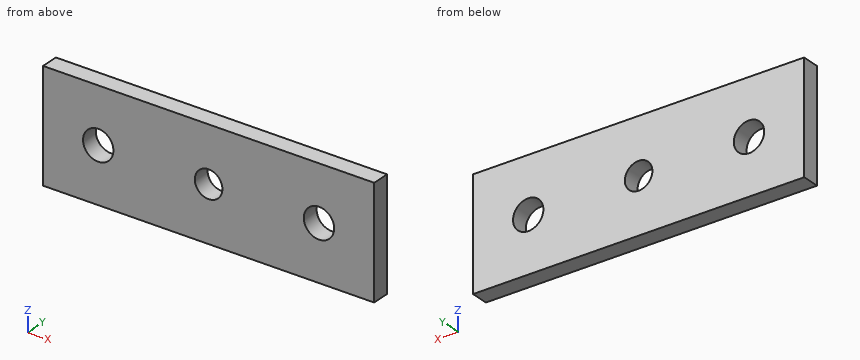
```python
from build123d import *

# Parameters (mm, degrees)
SKETCH1_W             = 60
SKETCH1_H             = 20
BOSS_EXTRUDE1_DEPTH   = 3.175
SKETCH4_R             = 2.75
CUT_EXTRUDE1_DEPTH    = 3.175
M6X1_0_TAPPED_HOLE1_D = 5


with BuildPart() as part:
    # Sketch1 → Boss-Extrude1 (new body)
    with BuildSketch(Plane(origin=(0, 0, 0), x_dir=(1, 0, 0), z_dir=(0, 1, 0))):
        with Locations((30, 10)):
            Rectangle(SKETCH1_W, SKETCH1_H)
    extrude(amount=BOSS_EXTRUDE1_DEPTH)

    # Sketch4 → Cut-Extrude1 (cut)
    with BuildSketch(Plane.XZ):
        with Locations((50, -10)):
            Circle(SKETCH4_R)
        with Locations((10, -10)):
            Circle(SKETCH4_R)
    extrude(amount=-CUT_EXTRUDE1_DEPTH, mode=Mode.SUBTRACT)

    # M6x1.0 Tapped Hole1 (through all)
    with Locations(Plane(origin=(30, 0, -10), x_dir=(0, 0, -1), z_dir=(0, -1, 0))):
        with Locations((0, 0)):
            Hole(M6X1_0_TAPPED_HOLE1_D / 2)


solid = part.part
```
Could you check a few things on this model? Use its own coordinates, in mm. Coordinates: 2 decimals unless noted, no trailing zeros. Write each loop counter-clockwise with the first axis right and the second up, starting at its lowest first coordinate (ties: lowest second). Pieces come first, ordered by that corner, then holes. Notation, with made-up numbers: M 33,-30.5 L 45,-30.5 A21 cw 45,-8.5 Z; hole C 30.5,46.5 d9. An arc over 180 degrees is marked long. Answer as CSV lines item,"result". Start each with the question number.
1) I want a section at A-A, the plane x = 50. Please give me the cut outline in (y, z) (3 decimals), and give its area (3 significant figures).
2) I want a section at D-D, the plane x = 30. Please give me the cut outline in (y, z) (3 decimals), and give its area (3 significant figures).
3) I want a section at C-C, the plane y = 0.6. Please give me the cut outline in (x, z).
4) I want a section at B-B, the plane z = -10. Please give me the cut outline in (x, y) (3 decimals), and give its area (3 significant figures).
5) Please list where these lines run through material, in increasing order: line 1 (Z direction, x = 50, y = 1.7); line 2 (Z direction, x = 28, y = 2.7). Write a range as from..to.
Data:
1,outline,"M 0,-20 L 3.175,-20 L 3.175,-12.75 L 0,-12.75 Z; M 0,-7.25 L 3.175,-7.25 L 3.175,0 L 0,0 Z"
1,area,"46.0 mm^2"
2,outline,"M 0,-20 L 3.175,-20 L 3.175,-12.5 L 0,-12.5 Z; M 0,-7.5 L 3.175,-7.5 L 3.175,0 L 0,0 Z"
2,area,"47.6 mm^2"
3,outline,"M 0,-20 L 60,-20 L 60,0 L 0,0 Z; hole C 10,-10 d5.5; hole C 30,-10 d5; hole C 50,-10 d5.5"
4,outline,"M 0,0 L 7.25,0 L 7.25,3.175 L 0,3.175 Z; M 12.75,0 L 27.5,0 L 27.5,3.175 L 12.75,3.175 Z; M 32.5,0 L 47.25,0 L 47.25,3.175 L 32.5,3.175 Z; M 52.75,0 L 60,0 L 60,3.175 L 52.75,3.175 Z"
4,area,"140 mm^2"
5,line 1,"z = -20..-12.75, -7.25..0"
5,line 2,"z = -20..-11.5, -8.5..0"
